Here's how the part is built. I have some questions about the finished solid (model axes, mm). A direction names the side the tool comes from. Round coordinates to 2 decimals unless told otherwise and drop trailing zeros. Loops run counter-clockwise (first coordinate to the right, second up) from the corner with the lowest first, then second, coordinate; pieces in that order, holes last. Notation, with made-up numbers: M 78,39 L 102,39 A7 cw 102,48 Z; hole C 72,26.25 d7. An arc over 180 degrees is marked long. Use a Markdown table: item, result.
from build123d import *

# Parameters (mm, degrees)
SKETCH1_W                                           = 190
SKETCH1_H                                           = 30
BOSS_EXTRUDE1_DEPTH                                 = 15
FILLET3_R                                           = 5
CBORE_FOR_M6_HEX_SOCKET_HEAD_CAP_SCREW1_D           = 6.6
CBORE_FOR_M6_HEX_SOCKET_HEAD_CAP_SCREW1_CBORE_D     = 13
CBORE_FOR_M6_HEX_SOCKET_HEAD_CAP_SCREW1_CBORE_DEPTH = 9


with BuildPart() as part:
    # Sketch1 → Boss-Extrude1 (new, symmetric)
    with BuildSketch(Plane.XY):
        Rectangle(SKETCH1_W, SKETCH1_H)
    extrude(amount=BOSS_EXTRUDE1_DEPTH, both=True)

    # Fillet3
    fillet3_edges = [part.edges().sort_by_distance(p)[0] for p in [
        (95, 0, 15),
        (0, 15, 15),
        (-95, 0, 15),
        (0, 15, -15),
        (95, 0, -15),
        (-95, 0, -15),
        (-95, 15, 0),
        (95, 15, 0),
    ]]
    fillet(fillet3_edges, radius=FILLET3_R)

    # CBORE for M6 Hex Socket Head Cap Screw1 (through all)
    with Locations(Plane(origin=(0, 15, 0), x_dir=(1, 0, 0), z_dir=(0, 1, 0))):
        with Locations((-80, 0), (80, 0)):
            CounterBoreHole(CBORE_FOR_M6_HEX_SOCKET_HEAD_CAP_SCREW1_D / 2, CBORE_FOR_M6_HEX_SOCKET_HEAD_CAP_SCREW1_CBORE_D / 2, CBORE_FOR_M6_HEX_SOCKET_HEAD_CAP_SCREW1_CBORE_DEPTH)


solid = part.part
1. Imagine slicing it at B-B, the plane x = 80. Write out the boundary of the cut face in (y, z), then the cut area to 3 significant figures.
Answer sheet:
| item | result |
|---|---|
| outline | M -15,-15 L 10,-15 A5 ccw 15,-10 L 15,-6.5 L 6,-6.5 L 6,-3.3 L -15,-3.3 Z; M -15,3.3 L 6,3.3 L 6,6.5 L 15,6.5 L 15,10 A5 ccw 10,15 L -15,15 Z |
| area | 634 mm2 |
2. For pin 1 Ø6 at (x, z) = (-80, 0) entering from -Y; pin 2 Ø6.5 at (x, z) = (-81, 2) entering from +Y, each with a flat end and sliding along its axis, tell me the tip position at first contact or that it passes through.
Answer sheet:
| item | result |
|---|---|
| pin 1 | through |
| pin 2 | y = 6 |
3. Which directions (+Z, -Z, +X, -X, +Y, -Y) give clear straight access to the entire face, cutting with the end or side of a thin tool? Please do faces 5 (the face through (77, 6, -2)), 6 (the face through (94, 13, 0)).
Answer sheet:
| item | result |
|---|---|
| face 5 | +Y |
| face 6 | +Z, -Z, +X, +Y |
4. Imagine slicing it at A-A, the plane z = 0. Write out the boundary of the cut face in (x, y), then the cut area to 3 significant figures.
Answer sheet:
| item | result |
|---|---|
| outline | M -95,-15 L -83.3,-15 L -83.3,6 L -86.5,6 L -86.5,15 L -90,15 A5 ccw -95,10 Z; M -76.7,-15 L 76.7,-15 L 76.7,6 L 73.5,6 L 73.5,15 L -73.5,15 L -73.5,6 L -76.7,6 Z; M 83.3,-15 L 95,-15 L 95,10 A5 ccw 90,15 L 86.5,15 L 86.5,6 L 83.3,6 Z |
| area | 5,180 mm2 |
5. We'd pull the mould along Z, two halves only. Please class faces 1 (the face through (-83, 6, -2)), 2 (the face through (-95, -3, 0)), 3 (the face through (-1, -2, -15)), 4 (the face through (-94, -2, 13)): +Z half, -Z half, draft (parallel to the pull), parting line (faces both ways), or undercut.
Answer sheet:
| item | result |
|---|---|
| face 1 | undercut |
| face 2 | draft |
| face 3 | -Z half |
| face 4 | +Z half |
6. Imagine slicing it at D-D, the plane z = 12.75. Write out the boundary of the cut face in (x, y).
Answer sheet:
| item | result |
|---|---|
| outline | M -94.18,-15 L 94.18,-15 L 94.18,10 A4.18 ccw 90,14.18 L -90,14.18 A4.18 ccw -94.18,10 Z |
7. Imagine slicing it at C-C, the plane y = -1. Write out the boundary of the cut face in (x, z).
Answer sheet:
| item | result |
|---|---|
| outline | M -95,-10 A5 ccw -90,-15 L 90,-15 A5 ccw 95,-10 L 95,10 A5 ccw 90,15 L -90,15 A5 ccw -95,10 Z; hole C -80,0 d6.6; hole C 80,0 d6.6 |
8. I need wall thicknesses on probe 1 along X at (y, z) = (-9.75, 2.5); probe 2 along X at (y, z) = (-5.5, 0.75); probe 3 along Z at (x, y) = (-80, 8.5). Which ranges of each line are inside material? Lowest first, please. Write a range as from..to.
Answer sheet:
| item | result |
|---|---|
| probe 1 | -95..-82.15, -77.85..77.85, 82.15..95 |
| probe 2 | -95..-83.21, -76.79..76.79, 83.21..95 |
| probe 3 | -15..-6.5, 6.5..15 |
